Verification items for the finished model (mm, model axes). A direction names the side the tool comes from. Give positions to 0.01 mm unless a question says otherwise; leave off trailing zeros. Write each loop counter-clockwise with the first axis right and the second up, starting at its lowest first coordinate (ties: lowest second). Pieces come first, ordered by that corner, then holes. Notation, with made-up numbers: (18, -6.75) -> (23, -6.75) arc R23 cw to (23, 24.25) -> close; hole circle Ø7 at (30, 62.25). An arc over 180 degrees is marked (long way). Use CSV: the item, a comma, the result in double quotes. Start each with the question number.
Autodesk Inventor part; units mm, degrees
ref_plane "Work Plane2" through (11.43, 0, 0) normal (1, 0, 0) x (0, 0, -1)
ref_plane "Work Plane1" through (-12.7, 0, 0) normal (1, 0, 0) x (0, 0, -1)
ref_plane "YZ Plane" through (0, 0, 0) normal (1, 0, 0) x (0, 1, 0)
sketch "Sketch1" plane through (0, 0, 0) normal (1, 0, 0) x (0, 1, 0)
  circle A0 centre (0, 0) radius 25.4
  dimension "d0" = 50.8
extrude "Extrusion1" add sketch "Sketch1" along normal blind 12.7
sketch "Sketch10" plane through (12.7, 0, 0) normal (1, 0, 0) x (0, 0, -1)
  point P0 (0, 0)
  point P1 (0, 0)
hole "Hole4" at (12.7, 0, 0) direction (-1, 0, 0) diameter 18.2563 depth 2.54
ref_plane "Work Plane2" through (11.43, 0, 0) normal (1, 0, 0) x (0, 0, -1)
hole "Hole1" at (11.43, 0, 0) direction (-1, 0, 0) diameter 13.0969 depth 4.7625
ref_plane "Work Plane1" through (-12.7, 0, 0) normal (1, 0, 0) x (0, 0, -1)
sketch "Sketch5" plane through (0, 0, 0) normal (1, 0, 0) x (0, 1, 0)
  line L0 (0, 9) -> (0, -9)
  circle A0 centre (0, 0) radius 25.4
  line L1 (-15.24, 0) -> (15.24, 0)
  line L2 (-15.24, 10.795) -> (-15.24, -10.795)
  dimension "d37" = 18
  dimension "d45" = 30.48
  dimension "d46" = 21.59
hole "Hole2" at (0, 0, -9) direction (1, 0, 0) diameter 2.159 depth 8.8646 tip angle 118
sketch "Sketch6" plane through (0, 0, 0) normal (-1, 0, 0) x (0, 0, 1)
  circle A0 centre (0, 0) radius 0.5715
  dimension "d34" = 1.143
hole "Hole5" at (0, 0, 0) direction (1, 0, 0) diameter 1 end through all
mirror "Mirror1" about plane through (0, 0, 0) normal (0, 0, 1) of "Hole2"
hole "Hole3" at (0, -15.24, 10.795) at (0, -15.24, -10.795) direction (1, 0, 0) diameter 2.9464 end through all counterbore diameter 4.826 counterbore depth 3.302
mirror "Mirror2" about plane through (0, 0, 0) normal (0, 1, 0) of "Hole3"
sketch "Sketch9" plane through (0, 0, 0) normal (0, 1, 0) x (-1, 0, 0)
  line L0 (-11.4554, -11.1125) -> (-12.7, -11.1125)
  line L1 (-12.7, -11.1125) -> (-12.7, -13.6525)
  line L2 (-12.7, -13.6525) -> (-11.4554, -13.6525)
  line L3 (-11.4554, -13.6525) -> (-11.4554, -11.1125)
  line L4 (2.54, 0) -> (-15.24, 0)
  line L5 (-12.7, 25.4) -> (-12.7, -25.4)
  point P0 (0, 0)
  dimension "d55" = 2.54
  dimension "d56" = 1.2446
  dimension "d59" = 11.1125
revolve "Revolution1" cut sketch "Sketch9" angle 360 about axis through (-10, 0, 0) along (1, 0, 0)
properties part number ".5 in hole" material "Aluminum 6061"
(1) Section check C-C on z = 5.5. Record the cut outline in (x, y), then the cut area to 3 significant figures.
(2) Go/stop test with flat-tipped pins: pin 1 (20 mm diameter, centred on y = -3, z = 1, fed in from +X); pin 2 (1 mm diameter, centred on x = 2, y = -18.5, fed in from +Z); pin 3 (2.5 mm diameter, centred on y = 15.24, z = 10.795, fed in from +X); pin 4 (5 mm diameter, centred on x = 10, z = -18, fed in from -Y). Record where each tip stops, or that it passes through.
(3) Section check D-D on x = 1.5. Record the cut outline in (y, z) (1 decimal).
(4) Thickness scan on line 1 (Z direction, x = 11.75, y = -5); line 2 (Z direction, x = 7.25, y = 15.24); line 3 (Z direction, x = 5.5, y = 14.5). Record the ranges inside material, lowest first. Write a range as from..to.
(5) Draft check along Z on faces 4 (the face through (3.302, -13.67, 11.3)), 5 (the face through (12.7, 11, -11)). Enter one of: released by +Z, released by -Z, zero draft, split by the parting line, or undercut.
(6) Set-up check for faces 1 (the face through (12.7, -8.3, 4.2)), 2 (the face through (3.302, 13.67, -11.3)), 3 (the face through (12.09, 3.34, -10.6)): record each of +Z, -Z, +X, -X, +Y, -Y from which the full face is reachable in a straight line by a thin tool's end or side.
(7) Section check B-B on y = 15.24. Record the cut outline in (x, z), then the cut area to 3 significant figures.
(8) Section check A-A on x = 8. Record the cut outline in (y, z) (1 decimal).
Data:
1,outline,"(0, -24.8) -> (12.7, -24.8) -> (12.7, -12.5) -> (11.46, -12.5) -> (11.46, -9.66) -> (12.7, -9.66) -> (12.7, -7.29) -> (10.16, -7.29) -> (10.16, -3.55) -> (6.67, -3.55) -> (6.67, 3.55) -> (10.16, 3.55) -> (10.16, 7.29) -> (12.7, 7.29) -> (12.7, 9.66) -> (11.46, 9.66) -> (11.46, 12.5) -> (12.7, 12.5) -> (12.7, 24.8) -> (0, 24.8) -> close"
1,area,"561 mm2"
2,pin 1,"stops at x = 12.7"
2,pin 2,"stops at z = 17.92"
2,pin 3,"passes through"
2,pin 4,"stops at y = -20.12"
3,outline,"circle Ø50.8 at (0, 0); hole circle Ø4.8 at (-15.2, -10.8); hole circle Ø4.8 at (-15.2, 10.8); hole circle Ø2.2 at (0, -9); hole circle Ø2.2 at (0, 9); hole circle Ø1 at (0, 0); hole circle Ø4.8 at (15.2, -10.8); hole circle Ø4.8 at (15.2, 10.8)"
4,line 1,"z = -24.9..-12.7, -9.92..-7.64, 7.64..9.92, 12.7..24.9"
4,line 2,"z = -20.32..-12.27, -9.32..9.32, 12.27..20.32"
4,line 3,"z = -20.85..-12.07, -9.52..9.52, 12.07..20.85"
5,face 4,"undercut"
5,face 5,"zero draft"
6,face 1,"+Z, -Z, +X, +Y, -Y"
6,face 2,"-X"
6,face 3,"+X"
7,outline,"(0, -20.32) -> (12.7, -20.32) -> (12.7, -12.27) -> (3.3, -12.27) -> (3.3, -13.21) -> (0, -13.21) -> close; (0, -8.38) -> (3.3, -8.38) -> (3.3, -9.32) -> (12.7, -9.32) -> (12.7, 9.32) -> (3.3, 9.32) -> (3.3, 8.38) -> (0, 8.38) -> close; (0, 13.21) -> (3.3, 13.21) -> (3.3, 12.27) -> (12.7, 12.27) -> (12.7, 20.32) -> (0, 20.32) -> close"
7,area,"429 mm2"
8,outline,"circle Ø50.8 at (0, 0); hole circle Ø2.9 at (-15.2, -10.8); hole circle Ø2.9 at (-15.2, 10.8); hole circle Ø13.1 at (0, 0); hole circle Ø2.2 at (0, -9); hole circle Ø2.2 at (0, 9); hole circle Ø2.9 at (15.2, -10.8); hole circle Ø2.9 at (15.2, 10.8)"
